Verification items for the finished model (mm, model axes). Face numbers are marked on the shaded views. A direction names the side the tool comes from. Round coordinates to 2 decimals unless told otherwise and drop trailing zeros. Write each loop counter-clockwise with the first axis right and the second up, starting at its lowest first coordinate (ties: lowest second). Pieces come first, ordered by that corner, then holes. Notation, with made-up numbers: M -8,2.25 L 31,2.25 A19 cw 31,28.25 Z; hole C 27.5,-28 d10. An arc over 180 degrees is marked long. Answer in a Markdown table with one row per item. Add a question column.
1. Set-up check for the marked faces 1 and 2: record each of +Z, -Z, +X, -X, +Y, -Y from which the full face is reachable in a straight line by a thin tool's end or side.
2. Material ranges on probe 1 along Y at (x, z) = (0, -4.7) (3 decimals); probe 2 along X at (y, z) = (4, -3.8); probe 3 along Z at (x, y) = (-5.25, -2), recorded low to high.
3. Sectioned sample at B-B on z = 10. Record the cut outline in (x, y), plus the area to 3 significant figures.
4. Go/stop test with flat-tipped pins: pin 1 Ø1.8 at (x, y) = (0, -8) entering from -Z; pin 2 Ø6 at (y, z) = (-4, 22) entering from +X; pin 3 Ø1.4 at (x, z) = (0, 29.869) entering from -Y. Record where each tip stops, or that it passes through.
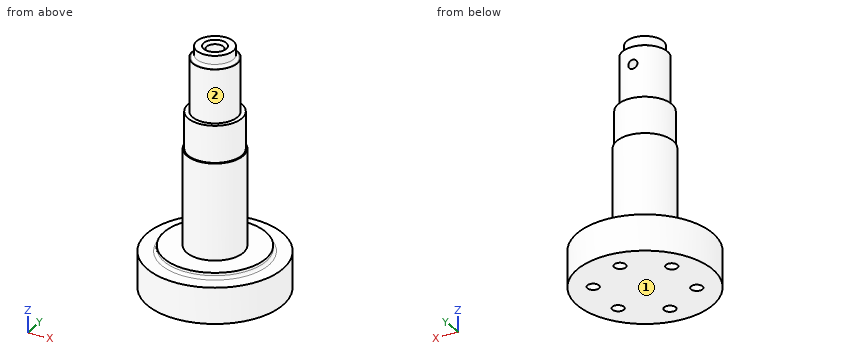
```python
from build123d import *

# Parameters (mm, degrees)
SKETCH4_W               = 0.8
SKETCH4_H               = 12
M2_5_TAPPED_HOLE1_D     = 2.05
M2_5_TAPPED_HOLE1_DEPTH = 5.35
M2_5_TAPPED_HOLE1_TIP   = 0.615882135
FILLET1_R               = 0.5
CHAMFER1_SIZE           = 0.5


with BuildPart() as part:
    # Sketch1 → Revolve1 (revolve)
    with BuildSketch(Plane(origin=(0, 0, 0), x_dir=(0, 0, -1), z_dir=(1, 0, 0))):
        with BuildLine():
            Line((0, 0), (-23.949, 0))
            Line((-23.949, 0), (-23.949, 1.5))
            Line((-23.949, 1.5), (-34.949, 1.5))
            Line((-34.949, 1.5), (-34.949, 3.25))
            Line((-34.949, 3.25), (-33.449, 3.25))
            ThreePointArc((-33.449, 3.25), (-33.095446609, 3.396446609), (-32.949, 3.75))
            Line((-32.949, 3.75), (-32.949, 3.96875))
            Line((-32.949, 3.96875), (-23.5, 3.96875))
            Line((-23.5, 3.96875), (-23.5, 4.7625))
            Line((-23.5, 4.7625), (-17, 4.7625))
            Line((-17, 4.7625), (-17, 5))
            Line((-17, 5), (0, 5))
            Line((0, 5), (0, 9))
            Line((0, 9), (1, 9))
            Line((1, 9), (1, 12))
            Line((1, 12), (7.35, 12))
            Line((7.35, 12), (7.35, 0))
            Line((7.35, 0), (0, 0))
        make_face()
    revolve(axis=Axis((0, 0, -7.35), (0, 0, 1)))

    # Sketch4 → M2 Tapped Hole1 (revolve, cut)
    with BuildSketch(Plane(origin=(0, 0, 29.869), x_dir=(0, 0, -1), z_dir=(1, 0, 0))):
        with Locations((0.4, 6)):
            Rectangle(SKETCH4_W, SKETCH4_H)
    revolve(axis=Axis((0, -6.35, 29.869), (0, 1, 0)), mode=Mode.SUBTRACT)

    # M2.5 Tapped Hole1
    with Locations(Plane(origin=(0, 0, -7.35), x_dir=(1, 0, 0), z_dir=(0, 0, -1))):
        with Locations((0, -8), (6.92820323, -4), (6.92820323, 4), (0, 8), (-6.92820323, 4), (-6.92820323, -4)):
            Hole(M2_5_TAPPED_HOLE1_D / 2, depth=M2_5_TAPPED_HOLE1_DEPTH)
            with Locations((0, 0, -(M2_5_TAPPED_HOLE1_DEPTH + M2_5_TAPPED_HOLE1_TIP / 2))):  # 118° drill point
                Cone(0, M2_5_TAPPED_HOLE1_D / 2, M2_5_TAPPED_HOLE1_TIP, mode=Mode.SUBTRACT)

    # Fillet1
    fillet1_edges = [part.edges().sort_by_distance(p)[0] for p in [
        (0, -9, -1),
    ]]
    fillet(fillet1_edges, radius=FILLET1_R)

    # Chamfer1
    chamfer1_edges = [part.edges().sort_by_distance(p)[0] for p in [
        (0, -1.5, 34.949),
    ]]
    chamfer(chamfer1_edges, length=CHAMFER1_SIZE)


solid = part.part
```
Geometry check:
| question | item | result |
|---|---|---|
| 1 | face 1 | -Z, +X, -X, +Y, -Y |
| 1 | face 2 | +Z |
| 2 | probe 1 | y = -12 to -9.025, -6.975 to 6.975, 9.025 to 12 |
| 2 | probe 2 | x = -11.31 to -7.95, -5.9 to 5.9, 7.95 to 11.31 |
| 2 | probe 3 | z = -7.35 to 0 |
| 3 | outline | C 0,0 d10 |
| 3 | area | 78.5 mm2 |
| 4 | pin 1 | stops at z = -1.92 |
| 4 | pin 2 | stops at x = 4.66 |
| 4 | pin 3 | stops at y = -3.97 |
